Work out the finished part from the listing and answer in its coordinate system (mm). A direction names the side the tool comes from. Give positions to 0.01 mm unless a question says otherwise; leave off trailing zeros. Write each loop counter-clockwise with the first axis right and the second up, starting at its lowest first coordinate (ties: lowest second). Pieces come first, ordered by that corner, then holes. Notation, with made-up numbers: (34.5, -7) - (65.5, -7) arc R19 cw to (65.5, 28) - close; hole circle Ø1 at (27, -27.75). An arc over 180 degrees is marked (long way). Write item = value, one per line.
from build123d import *

# Parameters (mm, degrees)
SKETCH_1_R               = 100
EXTRUDE_1_DEPTH          = 50
FILLET_1_R               = 25
SHELL_1_T                = -10
CUT_EXTRUDE_1_DEPTH      = 100
CUT_EXTRUDE_1_DEPTH_BACK = 100
SKETCH_7_R               = 9
SKETCH_8_R               = 8
EXTRUDE_2_DEPTH          = 10
SKETCH_9_W               = 19.636204252
SKETCH_9_H               = 30
EXTRUDE_3_DEPTH          = 3
SKETCH_10_R              = 8
EXTRUDE_4_DEPTH          = 10
SKETCH_11_W              = 19.636204252
SKETCH_11_H              = 25
EXTRUDE_5_DEPTH          = 3


with BuildPart() as part:
    # Sketch 1 → Extrude 1 (new body)
    with BuildSketch(Plane(origin=(0, 0, 0), x_dir=(1, 0, 0), z_dir=(0, 1, 0))):
        with Locations(Location((0, 0, 0), (0, 0, 270))):
            Circle(SKETCH_1_R)
    extrude(amount=EXTRUDE_1_DEPTH)

    # Fillet 1
    fillet_1_edges = [part.edges().sort_by_distance(p)[0] for p in [
        (0, 50, -100),
    ]]
    fillet(fillet_1_edges, radius=FILLET_1_R)

    # Shell 1
    shell_1_openings = [part.faces().sort_by_distance(p)[0] for p in [
        (0, 0, 0),
    ]]
    offset(amount=SHELL_1_T, openings=shell_1_openings, kind=Kind.INTERSECTION)

    # Sketch 7 → Cut-Extrude 1 (cut, two sides: drawn at the far end of the back side and taken through both)
    with BuildSketch(Plane(origin=(0, 0, 0), x_dir=(0, 0, -1), z_dir=(1, 0, 0)).offset(-CUT_EXTRUDE_1_DEPTH_BACK)):
        with Locations(Location((0, 11.380292073, 0), (0, 0, 180))):
            Circle(SKETCH_7_R)
    extrude(amount=CUT_EXTRUDE_1_DEPTH + CUT_EXTRUDE_1_DEPTH_BACK, mode=Mode.SUBTRACT)



with BuildPart() as body_2:
    # Sketch 8 → Extrude 2 (new body)
    with BuildSketch(Plane(origin=(90, 0, 0), x_dir=(0, 0, -1), z_dir=(1, 0, 0))):
        with Locations((0, 11.380292073)):
            Circle(SKETCH_8_R)
    extrude(amount=EXTRUDE_2_DEPTH)


with BuildPart() as part_1:
    add(part.part)

    add(body_2.part)  # Extrude 3 merges body 2
    # Sketch 9 → Extrude 3 (add)
    with BuildSketch(Plane(origin=(90, 0, 0), x_dir=(0, 0, -1), z_dir=(1, 0, 0))):
        with Locations((0, 16.380292073)):
            Rectangle(SKETCH_9_W, SKETCH_9_H)
    extrude(amount=-EXTRUDE_3_DEPTH)



with BuildPart() as body_2_2:
    # Sketch 10 → Extrude 4 (new body)
    with BuildSketch(Plane(origin=(-90, 0, 0), x_dir=(0, 0, -1), z_dir=(1, 0, 0))):
        with Locations((0, 11.380292073)):
            Circle(SKETCH_10_R)
    extrude(amount=-EXTRUDE_4_DEPTH)


with BuildPart() as part_2:
    add(part_1.part)

    add(body_2_2.part)  # Extrude 5 merges body 2 2
    # Sketch 11 → Extrude 5 (add)
    with BuildSketch(Plane(origin=(-90, 0, 0), x_dir=(0, 0, -1), z_dir=(1, 0, 0))):
        with Locations((0, 14.380292073)):
            Rectangle(SKETCH_11_W, SKETCH_11_H)
    extrude(amount=EXTRUDE_5_DEPTH)


solid = part_2.part
1. Find section C-C, the plane x = 0. Give the vertices of the cut face in (y, z).
Solution:
outline = (0, -100) - (25, -100) arc R25 ccw to (50, -75) - (50, 75) arc R25 ccw to (25, 100) - (0, 100) - (0, 90) - (25, 90) arc R15 cw to (40, 75) - (40, -75) arc R15 cw to (25, -90) - (0, -90) - close
2. Given pin 1 (0.7 mm diameter, centred on x = 88.5, y = 21.5, fed in from +Z); pin 2 (2 mm diameter, centred on y = 11.5, z = -66.5, fed in from +X); pin 3 (2 mm diameter, centred on y = 25, z = 63, fed in from +X); pin 4 (10 mm diameter, centred on x = -75.5, z = -74.5, fed in from +Y), each flat-ended and moving along its own axis, determine where each tip first touches the part or whether it passes through.
Solution:
pin_1 = 47.22
pin_2 = 75.56
pin_3 = 78.46
pin_4 = through
3. Straight lines are drawn through the part: line 1 (X direction, y = 8.75, z = 0); line 2 (Y direction, x = -97, z = 0); line 3 (Y direction, x = -94, z = 0). For each, find the intervals that lie inside material, in ascending order.
Solution:
line_1 = -100 to -87, 87 to 100
line_2 = 0 to 2.38, 3.38 to 19.38, 20.38 to 36.87
line_3 = 0 to 2.38, 3.38 to 19.38, 20.38 to 41.25
4. For a pull along Z with two mould halves and no side action, classify faces 4 (the flat face through (-100, 11, 0)), 5 (the flat face through (1, 40, -1)), 6 (the cylindrical face through (94.93, 19.312, 1.041)), 7 (the cylindrical face through (30.04, 12.32, 95.38)) as pulls with the +Z half, pulls with the -Z half, needs draft (parallel to the pull), parting line crosses it, or undercut.
Solution:
face_4 = needs draft
face_5 = undercut
face_6 = undercut
face_7 = parting line crosses it
5. A tool of negligible diameter and unlimited length cuts with its end or side. For faces 1 (the flat face through (87, 17, 0)), 2 (the cylindrical face through (-94.93, 19.312, 1.041)), 3 (the cylindrical face through (94.93, 2.457, -1.172)), from which of +Z, -Z, +X, -X, +Y, -Y can it reach the whole face along a straight path? Write none if from no direction.
Solution:
face_1 = -Y
face_2 = -X
face_3 = +X
6. Find section B-B, the plane y = 6. Give the vertices of the cut face in (x, z), then the cut area to 3 significant figures.
Solution:
outline = (-100, -5.92) - (-90, -5.92) - (-90, -7.21) - (-99.74, -7.21) arc R100 ccw to (99.74, -7.21) - (90, -7.21) - (90, -5.92) - (100, -5.92) - (100, 5.92) - (90, 5.92) - (90, 7.21) - (99.74, 7.21) arc R100 ccw to (-99.74, 7.21) - (-90, 7.21) - (-90, 5.92) - (-100, 5.92) - close; hole (-89.46, -9.82) arc R90 ccw to (89.46, -9.82) - (87, -9.82) - (87, 9.82) - (89.46, 9.82) arc R90 ccw to (-89.46, 9.82) - (-87, 9.82) - (-87, -9.82) - close
area = 6,030 mm^2
